Can you work these out from the drawing? Everything is in mm from the part's minimum corner. A direction names the side the tool comes from. Round coordinates to 2 decimals unless told otherwise and drop trailing zeros. Loops run counter-clockwise (first coordinate to the right, second up) from the corner with the lowest first, then second, coordinate; pieces in that order, holes last. Notation, with made-up numbers: M 64.25,63.5 L 109.25,63.5 A19 ccw 109.25,78.5 Z; hole C 32.25,83.25 d4. An arc over 180 degrees is marked long. Use a Markdown table: item, result.
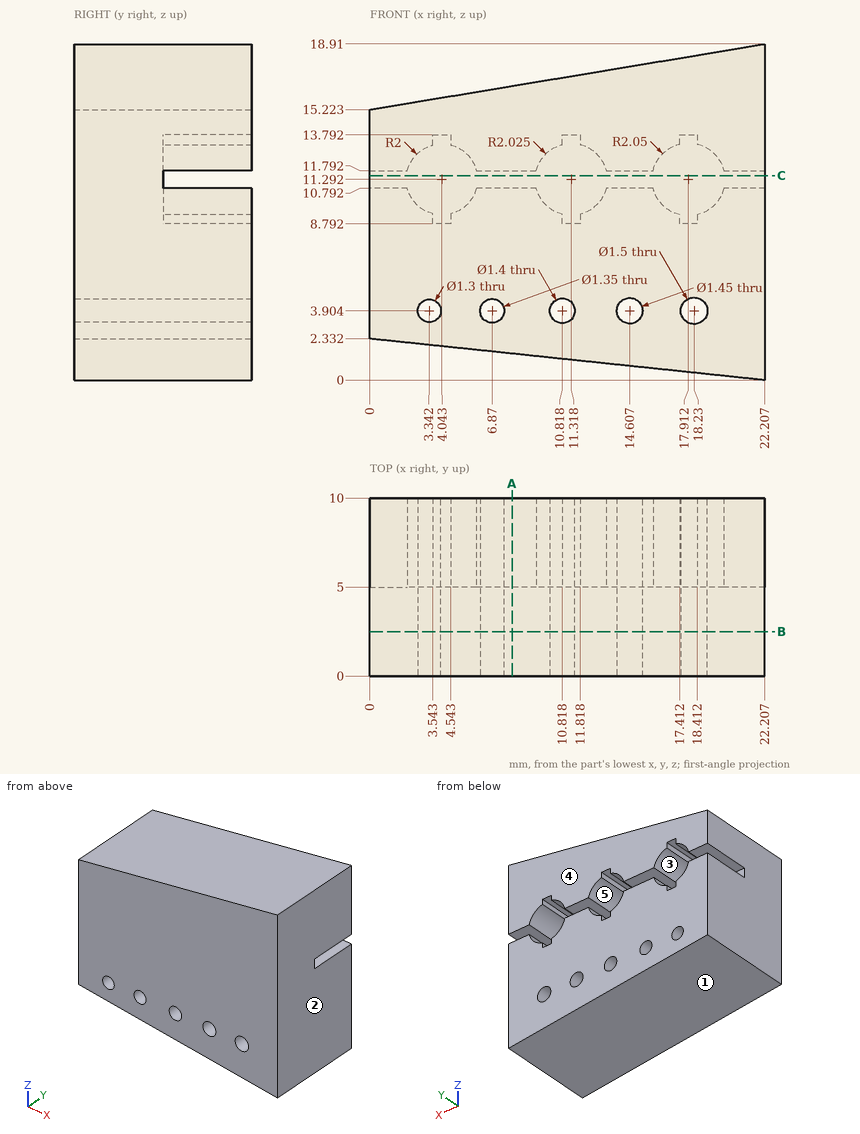
1. We'd pull the mould along Z, two halves only. Please class the marked faces 1, 2 and 3: +Z half, -Z half, draft (parallel to the pull), parting line (faces both ways), or undercut.
Answer sheet:
| item | result |
|---|---|
| face 1 | -Z half |
| face 2 | draft |
| face 3 | undercut |
2. Imagine slicing it at B-B, the plane y = 2.5. State how many separate pieces and enclosed holes the cut face has, then the cut area to 3 significant figures.
Answer sheet:
| item | result |
|---|---|
| separate pieces | 1 |
| enclosed holes | 5 |
| area | 345 mm2 |
3. I need wall thicknesses on probe 1 along X at (y, z) = (8, 12) (1 decimal); probe 2 along Z at (x, y) = (14.25, 6.25) (1 decimal); probe 3 along Z at (x, y) = (10.25, 8.5) (1 decimal). Which ranges of each line are inside material? Lowest first, please. Write a range as from..to.
Answer sheet:
| item | result |
|---|---|
| probe 1 | 0..2.2, 5.9..9.4, 13.2..16, 19.8..22.2 |
| probe 2 | 0.8..3.3, 4.5..10.8, 11.8..17.6 |
| probe 3 | 1.3..3.5, 4.3..9.6, 13..16.9 |
4. For pin 1 Ø1.5 at (x, y) = (6.5, 6) entering from -Z; pin 2 Ø1.2 at (x, z) = (6.87, 3.9) entering from -Y; pin 3 Ø0.8 at (x, y) = (4.5, 8) entering from -Z; pin 4 Ø2 at (x, y) = (4, 4) entering from +Z, each with a flat end and sliding along its axis, tell me the tip position at first contact or that it passes through.
Answer sheet:
| item | result |
|---|---|
| pin 1 | z = 1.57 |
| pin 2 | through |
| pin 3 | z = 1.82 |
| pin 4 | z = 16.05 |
5. Imagine slicing it at C-C, the plane z = 11.5. Write out the boundary of the cut face in (x, y).
Answer sheet:
| item | result |
|---|---|
| outline | M 0,0 L 22.21,0 L 22.21,5 L 0,5 Z |
6. Imagine slicing it at A-A, the plane x = 8. Write out the boundary of the cut face in (y, z).
Answer sheet:
| item | result |
|---|---|
| outline | M 0,1.49 L 10,1.49 L 10,10.79 L 5,10.79 L 5,11.79 L 10,11.79 L 10,16.55 L 0,16.55 Z |
7. Which directions (+Z, -Z, +X, -X, +Y, -Y) give clear straight access to the entire face, cutting with the end or side of a thin tool? Please do the marked faces 4 and 5.
Answer sheet:
| item | result |
|---|---|
| face 4 | +Z, -Z, +X, -X, +Y |
| face 5 | +Y |
